Read the model definition and answer for the solid it produces. Units are mm, in the model's axes. Coordinates: 2 decimals unless noted, no trailing zeros. Loops run counter-clockwise (first coordinate to the right, second up) from the corner with the lowest first, then second, coordinate; pieces in that order, holes last. Notation, with made-up numbers: M 5.25,15.25 L 53.25,15.25 A16 ccw 53.25,29.25 Z; hole C -32.75,75.5 d1. An arc over 180 degrees is marked long. Put each result on its own line as item: value.
from build123d import *

# Parameters (mm, degrees)
ESBO_O1_W                = 143.01
ESBO_O1_H                = 54.05
RESSALTO_EXTRUS_O1_DEPTH = 6.35
ESBO_O2_R                = 2.755
ESBO_O2_R_2              = 2.755565393
ESBO_O2_R_3              = 2.735691737
CORTE_EXTRUS_O1_DEPTH    = 6.35
ESBO_O3_R                = 15.995
ESBO_O3_R_2              = 10
CORTE_EXTRUS_O2_DEPTH    = 10
ESBO_O4_W                = 143.01
ESBO_O4_H                = 3.42
RESSALTO_EXTRUS_O2_DEPTH = 6.35
ESBO_O5_R                = 16
CORTE_EXTRUS_O3_DEPTH    = 10
ESBO_O6_R                = 1.5
CORTE_EXTRUS_O4_DEPTH    = 15


with BuildPart() as part:
    # Esboço1 → Ressalto-extrusão1 (new body)
    with BuildSketch(Plane.XY):
        Rectangle(ESBO_O1_W, ESBO_O1_H)
    extrude(amount=RESSALTO_EXTRUS_O1_DEPTH)

    # Esboço2 → Corte-extrusão1 (cut)
    with BuildSketch(Plane(origin=(0, 0, 0), x_dir=(-1, 0, 0), z_dir=(0, 0, -1))):
        with Locations((-44.463136928, 23.291850449)):
            Circle(ESBO_O2_R)
        with Locations((-65.913136928, 1.841850449)):
            Circle(ESBO_O2_R_2)
        with Locations((-44.463136928, -19.608149551)):
            Circle(ESBO_O2_R_3)
        with Locations((-23.013136928, 1.841850449)):
            Circle(ESBO_O2_R)
        with Locations((23.016863072, 1.841850449)):
            Circle(ESBO_O2_R)
        with Locations((44.466863072, -19.608149551)):
            Circle(ESBO_O2_R)
        with Locations((65.916863072, 1.841850449)):
            Circle(ESBO_O2_R)
        with Locations((44.466863072, 23.291850449)):
            Circle(ESBO_O2_R)
    extrude(amount=-CORTE_EXTRUS_O1_DEPTH, mode=Mode.SUBTRACT)

    # Esboço3 → Corte-extrusão2 (cut)
    with BuildSketch(Plane(origin=(0, 0, 0), x_dir=(-1, 0, 0), z_dir=(0, 0, -1))):
        with Locations((-44.463136928, 1.841850449)):
            Circle(ESBO_O3_R)
        with Locations((0.001863072, 1.841850449)):
            Circle(ESBO_O3_R_2)
        with Locations((44.466863072, 1.841850449)):
            Circle(ESBO_O3_R)
    extrude(amount=-CORTE_EXTRUS_O2_DEPTH, mode=Mode.SUBTRACT)

    # Esboço4 → Ressalto-extrusão2 (add)
    with BuildSketch(Plane.XY):
        with Locations((0, 28.735)):
            Rectangle(ESBO_O4_W, ESBO_O4_H)
    extrude(amount=RESSALTO_EXTRUS_O2_DEPTH)

    # Esboço5 → Corte-extrusão3 (cut)
    with BuildSketch(Plane.XY.offset(6.35)):
        with Locations((-0.001863072, 1.841850449)):
            Circle(ESBO_O5_R)
    extrude(amount=-CORTE_EXTRUS_O3_DEPTH, mode=Mode.SUBTRACT)

    # Esboço6 → Corte-extrusão4 (cut)
    with BuildSketch(Plane(origin=(0, 30.445, 0), x_dir=(1, 0, 0), z_dir=(0, 1, 0))):
        with Locations(Location((56.423186497, -3.175, 0), (0, 0, 270))):
            Circle(ESBO_O6_R)
        with Locations(Location((26.423186497, -3.175, 0), (0, 0, 270))):
            Circle(ESBO_O6_R)
        with Locations(Location((-26.423186497, -3.175, 0), (0, 0, 90))):
            Circle(ESBO_O6_R)
        with Locations(Location((-56.423186497, -3.175, 0), (0, 0, 90))):
            Circle(ESBO_O6_R)
    extrude(amount=-CORTE_EXTRUS_O4_DEPTH, mode=Mode.SUBTRACT)


solid = part.part
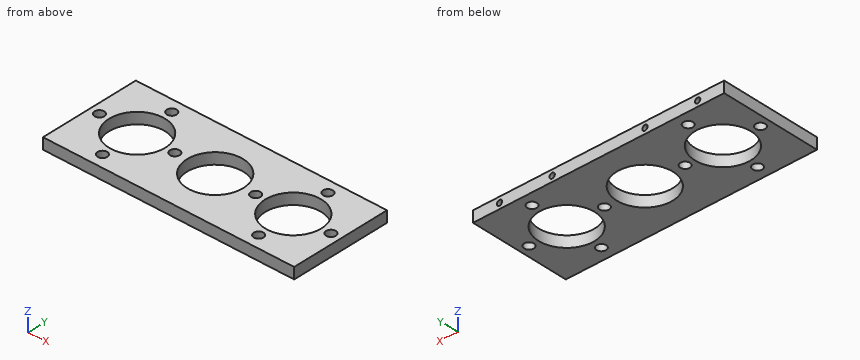
1) Find section B-B, the plane x = -40. Write down the section's boundary in (y, z) (3 decimals).
Answer list:
outline: M -27.025,0 L -13.517,0 L -13.517,6.35 L -27.025,6.35 Z; M 17.2,0 L 30.445,0 L 30.445,6.35 L 17.2,6.35 Z
2) Find section A-A, the plane y = 13.5. Write down the section's boundary in (x, z) (3 decimals), plus the area to 3 significant figures.
Answer list:
outline: M -71.505,0 L -55.418,0 L -55.418,6.35 L -71.505,6.35 Z; M -33.516,0 L -10.96,0 L -10.96,6.35 L -33.516,6.35 Z; M 10.957,0 L 33.512,0 L 33.512,6.35 L 10.957,6.35 Z; M 55.414,0 L 71.505,0 L 71.505,6.35 L 55.414,6.35 Z
area: 491 mm^2
3) Find section C-C, the plane z = 3.25. Count the separate pieces of the cut face and the enclosed holes in it, plus the area to 3 significant figures.
Answer list:
separate pieces: 1
enclosed holes: 11
area: 5,440 mm^2
4) Straight lines are drawn through the part: line 1 (X direction, y = 26.5, z = 3) (3 decimals); line 2 (X direction, y = -6.5, z = 2.75) (3 decimals); line 3 (X direction, y = -4.5, z = 2.75) (3 decimals). For each, find the intervals that lie inside material, in ascending order. Write a range as [from, to].
Answer list:
line 1: x = [-71.505, -57.913], [-54.933, -27.913], [-24.933, 24.933], [27.913, 54.933], [57.913, 71.505]
line 2: x = [-71.505, -58.114], [-30.819, -13.655], [13.651, 30.816], [58.111, 71.505]
line 3: x = [-71.505, -59.151], [-29.783, -14.691], [14.688, 29.779], [59.147, 71.505]
5) Find section D-D, the plane y = 7.5. Write down the section's boundary in (x, z) (3 decimals), plus the area to 3 significant figures.
Answer list:
outline: M -71.505,0 L -59.428,0 L -59.428,6.35 L -71.505,6.35 Z; M -29.506,0 L -14.968,0 L -14.968,6.35 L -29.506,6.35 Z; M 14.964,0 L 29.502,0 L 29.502,6.35 L 14.964,6.35 Z; M 59.424,0 L 71.505,0 L 71.505,6.35 L 59.424,6.35 Z
area: 338 mm^2
6) Given pin 1 Ø0.9 at (x, z) = (57, 3.5) entering from +Y (3 decimals); pin 2 Ø4.5 at (x, y) = (44.46, 23.29) entering from +Z, each flat-ended and moving along its own axis, determine where each tip first touches the part or whether it passes through.
Answer list:
pin 1: stops at y = 15.445
pin 2: passes through
